For this review, use the dimensioned drawing (mm, ordinates from the lowest corner) and the shaded views. A direction names the side the tool comes from. Give positions to 0.01 mm unless a question says otherwise; leave off trailing zeros. Order: outer loops, then holes, each group sorted by start corner. A loop starts at its lowest first (then second) coordinate and runs counter-clockwise, first axis right, second up.
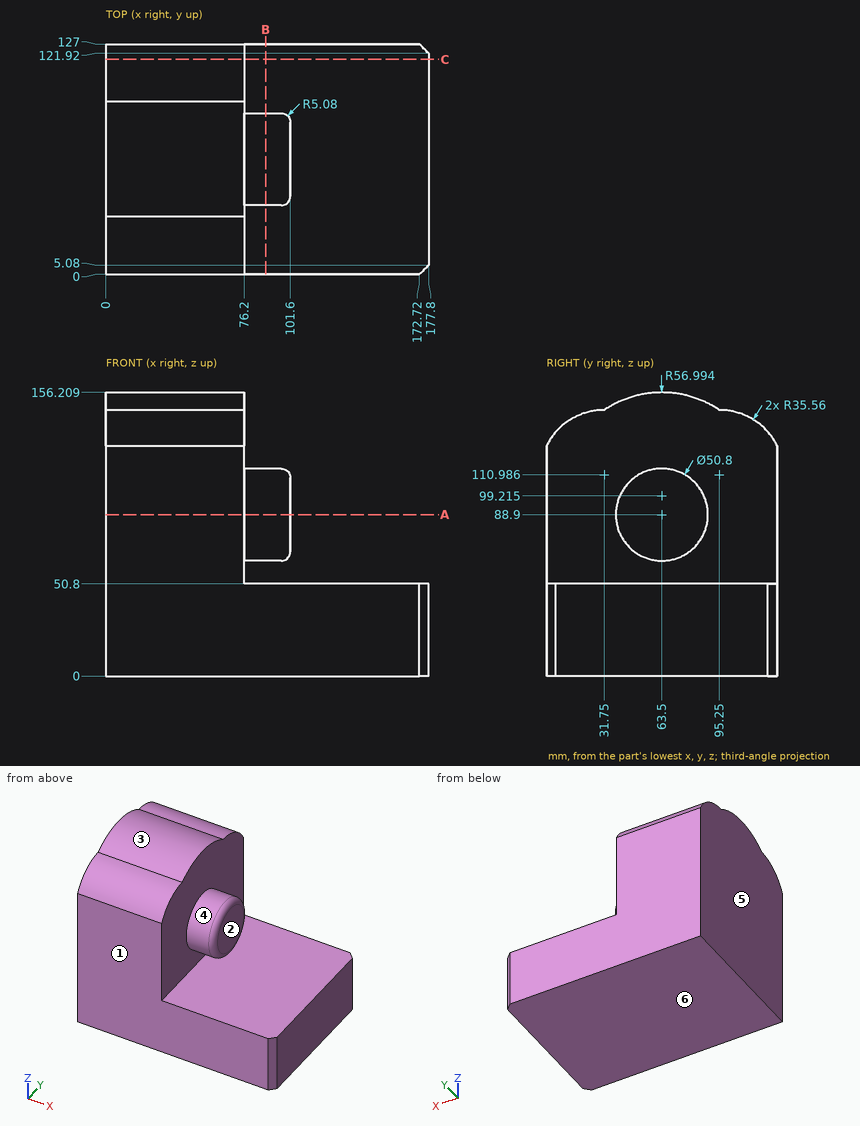
1. Take a section at A-A (z = 88.9). State the section outline as (x, y) points, then the cut area to 3 significant figures.
Recorded:
outline: (0, 0) - (76.2, 0) - (76.2, 38.1) - (96.52, 38.1) arc R5.08 ccw to (101.6, 43.18) - (101.6, 83.82) arc R5.08 ccw to (96.52, 88.9) - (76.2, 88.9) - (76.2, 127) - (0, 127) - close
area: 11,000 mm2
2. Take a section at C-C (y = 118.5). State the section outline as (x, z) points, then the cut area to 3 significant figures.
Recorded:
outline: (0, 0) - (177.8, 0) - (177.8, 50.8) - (76.2, 50.8) - (76.2, 137.89) - (0, 137.89) - close
area: 15,700 mm2
3. For line 1 along X through (y, z) = (11, 94); line 2 along X through (y, z) = (53.5, 79.5); line 3 along Z through (x, y) = (112, 9), list the stretches that pass through material, from the lowest coordinate up.
Recorded:
line 1: x = 0 to 76.2
line 2: x = 0 to 101.6
line 3: z = 0 to 50.8
4. For pin 1 (4 mm diameter, centred on x = 97, y = 96, fed in from +Z); pin 2 (1.5 mm diameter, centred on y = 106, z = 97, fed in from +X); pin 3 (6 mm diameter, centred on x = 36, y = 92, fed in from +Z) (1 decimal), all flat-tipped, find the tip position at first contact; note any pin that passes through.
Recorded:
pin 1: stops at z = 50.8
pin 2: stops at x = 76.2
pin 3: stops at z = 150.2
5. Take a section at B-B (x = 88). State the section outline as (y, z) points.
Recorded:
outline: (0, 0) - (127, 0) - (127, 50.8) - (0, 50.8) - close; circle Ø50.8 at (63.5, 88.9)
6. Machinability: for the marked faces 1 and 2, which of the approach directions +Z, -Z, +X, -X, +Y, -Y give a long, thin tool a straight path to every point of the face, cutting with its end or side? Answer none if there is none.
Recorded:
face 1: +Z, -Z, +X, -X, -Y
face 2: +Z, +X, +Y, -Y
7. Draft analysis for pull direction Z (two halves, no side actions). For the marked faces 3, 4, 5 and 6, state which applies: pulls with the +Z half, pulls with the -Z half, needs draft (parallel to the pull), parting line crosses it, or undercut.
Recorded:
face 3: pulls with the +Z half
face 4: undercut
face 5: needs draft
face 6: pulls with the -Z half
